The listing builds one solid part. Answer for the finished solid, in the listing's coordinates (mm). A direction names the side the tool comes from. Coordinates: 2 decimals unless noted, no trailing zeros. Loops run counter-clockwise (first coordinate to the right, second up) from the corner with the lowest first, then second, coordinate; pieces in that order, holes last. Notation, with made-up numbers: (78.25, 54) - (87.25, 54) arc R6 ccw to (87.25, 65) - close; hole circle Ø5 at (18.5, -35.75). An arc over 180 degrees is marked (long way). Return JSON: item names as keys, results as strings. Group by question number.
1. Section D-D (y = -12) is taken. Write down the section's boundary in (x, z).
2. Which of the six approach directions +Z, -Z, +X, -X, +Y, -Y give full straight-line access (tool end or side, diameter ignored) to faces 1 (the face through (23, -10, 12)), 2 (the face through (-20, -9, 36)), 3 (the face through (-23.04, 4.21, 38.35))?
3. The mould has two halves that part along Z. Classify faces 4 (the face through (-22.958, 12.843, 15.032)), 5 (the face through (0, -35, 3)), 6 (the face through (-22.958, 11.903, 34.802)), 7 (the face through (0, -10, 0)): pulls with the +Z half, pulls with the -Z half, needs draft (parallel to the pull), parting line crosses it, or undercut.
4. Section A-A (z = 25) is taken. Write down the section's boundary in (x, y), and give its area (3 significant figures).
5. Each of these flat-tipped pins is pushed along its axis until it touches: P1, Ø6.5, axis at x = 24, z = 27, coming from the -Y side; P2, Ø8, axis at y = -28, z = 13.5, coming from the +X side; P3, Ø1.8, axis at x = 22, y = -9.5, coming from the +Z side. Where does it stop, or does it pass through?
6. Section B-B (x = -21.5) is taken. Write down the section's boundary in (y, z).
7. Section C-C (z = 7) is taken. Write down the section's boundary in (x, y), and give its area (3 significant figures).
8. Find the intervals of material crossed by line 1 along Y through (x, z) = (-22.3, 37); line 2 along Y through (x, z) = (-22, 25); line 3 along Z through (x, y) = (-22.5, -12.5), in increasing order.
Autodesk Inventor part; units mm, degrees
ref_plane "YZ Plane" through (0, 0, 0) normal (1, 0, 0) x (0, 1, 0)
ref_plane "XZ Plane" through (0, 0, 0) normal (0, 1, 0) x (-1, 0, 0)
ref_plane "XY Plane" through (0, 0, 0) normal (0, 0, 1) x (1, 0, 0)
sketch "スケッチ1" plane through (0, 0, 0) normal (0, 0, 1) x (1, 0, 0)
  circle A0 centre (0, 0) radius 14
  line L0 (-12, -12) -> (12, -12)
  line L1 (12, -12) -> (12, 12)
  line L2 (12, 12) -> (-12, 12)
  line L3 (-12, 12) -> (-12, -12)
  line L4 (-12, -12) -> (12, 12) construction
  line L5 (12, -12) -> (-12, 12) construction
  circle A1 centre (-12, 12) radius 1.45
  circle A2 centre (12, 12) radius 1.45
  circle A3 centre (-12, -12) radius 1.45
  circle A4 centre (12, -12) radius 1.45
  line L6 (-20, -15) -> (20, -15)
  line L7 (20, -15) -> (20, 15)
  line L8 (20, 15) -> (-20, 15)
  line L9 (-20, 15) -> (-20, -15)
  line L10 (-20, -15) -> (20, 15) construction
  line L11 (20, -15) -> (-20, 15) construction
  dimension "d0" = 24
  dimension "d1" = 24
  dimension "d2" = 28
  dimension "d3" = 2.9
  dimension "d4" = 2.9
  dimension "d5" = 2.9
  dimension "d6" = 2.9
  dimension "d7" = 30
  dimension "d8" = 40
extrude "押し出し1" add sketch "スケッチ1" along normal blind 6 contours A0 L1 | L1 A0 L0 L3 L2 | A0 L2 A2 L1 | L1 A4 L0 A0 | L2 A0 | A2 L2 L1 | L1 L2 A2 | A0 L0 | A4 L0 L1 | L1 L0 A4 | A0 L3 A1 L2 | L0 A3 L3 A0 | L3 A0 | A1 L3 L2 | L2 L3 A1 | A3 L3 L0 | L0 L3 A3 | L9 L8 L7 L6
sketch "スケッチ3" plane through (0, 0, 0) normal (0, 0, -1) x (-1, 0, 0)
  line L0 (-20, -15) -> (-20, 15)
  line L1 (20, 15) -> (20, -15)
  line L2 (-20, 15) -> (-26, 15)
  line L3 (-26, 15) -> (-26, -15)
  line L4 (-26, -15) -> (-20, -15)
  line L5 (-20, -15) -> (-20, 15)
  line L6 (20, -15) -> (26, -15)
  line L7 (26, -15) -> (26, 15)
  line L8 (26, 15) -> (20, 15)
  line L9 (20, 15) -> (20, -15)
  dimension "d16" = 6
  dimension "d17" = 6
extrude "押し出し2" add sketch "スケッチ3" against normal blind 55
sketch "スケッチ7" plane through (-26, -15, 0) normal (0, -1, 0) x (1, 0, 0)
  line L0 (52, 0) -> (0, 0)
  line L1 (52, 0) -> (52, 55)
  line L2 (6, 6) -> (46, 6)
  line L3 (0, 0) -> (0, 55)
  line L4 (52, 0) -> (0, 0)
  line L5 (0, 0) -> (52, 0)
  line L6 (52, 0) -> (52, 6)
  line L7 (52, 6) -> (0, 6)
  line L8 (0, 6) -> (0, 0)
  point P0 (26, 0)
  point P1 (0, 6)
extrude "押し出し5" add sketch "スケッチ7" along normal blind 20
sketch "スケッチ8" plane through (0, 0, 0) normal (0, 0, -1) x (-1, 0, 0)
  line L0 (-26, 15) -> (26, 15)
  line L1 (26, -35) -> (26, 15)
  circle A0 centre (-1.5, -10.4) radius 25.65
  circle A1 centre (21.5, -30.4) radius 1.6
  circle A2 centre (-21.5, 7.6) radius 1.6
  point P0 (0, 0)
  dimension "d29" = 51.3
  dimension "d30" = 3.2
  dimension "d31" = 3.2
  dimension "d34" = 20
  dimension "d35" = 18
  dimension "d36" = 23
  dimension "d37" = 20
  dimension "d38" = 45.4
  dimension "d39" = 4.5
hole "穴1" at (-21.5, -30.4, 0) at (21.5, 7.6, 0) direction (0, 0, 1) diameter 4.4 depth 5
sketch "Sketch10" plane through (-26, -15, 55) normal (-1, 0, 0) x (0, 0, 1)
  line L0 (-55, -20) -> (-55, 30)
  line L1 (-49, -20) -> (-55, -20)
  line L2 (-49, 0) -> (-49, -20)
  line L3 (-49, 0) -> (0, 0)
  line L4 (0, 30) -> (0, 0)
  line L5 (-55, 30) -> (0, 30)
  circle A0 centre (-30, 15) radius 14
  point P0 (-55, 15)
  dimension "d58" = 28
  dimension "d59" = 15
  dimension "d60" = 25
extrude "Extrusion7" cut sketch "Sketch10" against normal blind 10 contours A0
sketch "Sketch11" plane through (-26, -15, 55) normal (-1, 0, 0) x (0, 0, 1)
  circle A0 centre (-30, 15) radius 14
  line L0 (-18, 27) -> (-42, 27)
  line L1 (-42, 27) -> (-42, 3)
  line L2 (-42, 3) -> (-18, 3)
  line L3 (-18, 3) -> (-18, 27)
  line L4 (-18, 27) -> (-42, 3) construction
  line L5 (-42, 27) -> (-18, 3) construction
  point P0 (-55, 15)
  dimension "d63" = 24
  dimension "d64" = 24
hole "Hole2" at (-26, -12, 37) at (-26, 12, 37) at (-26, 12, 13) at (-26, -12, 13) direction (1, 0, 0) diameter 4.4 depth 8.8 tip angle 118
sketch "スケッチ12" plane through (26, -15, 55) normal (1, 0, 0) x (0, 0, -1)
  line L0 (0, 0) -> (0, 30)
  line L1 (49, 0) -> (0, 0)
  line L2 (49, 0) -> (49, -20)
  line L3 (49, 0) -> (0, 0)
  line L4 (0, 0) -> (43, 0)
  line L5 (43, 0) -> (43, 10)
  line L6 (43, 10) -> (0, 10)
  line L7 (0, 10) -> (0, 0)
  point P0 (55, 15)
  point P1 (0, 10)
  dimension "d75" = 10
  dimension "d76" = 6
extrude "押し出し8" cut sketch "スケッチ12" against normal blind 10
sketch "スケッチ13" plane through (-26, -15, 6) normal (0, -1, 0) x (1, 0, 0)
  line L0 (0, 0) -> (6, 0)
  line L1 (6, 0) -> (6, 49)
  line L2 (0, 49) -> (6, 49)
  line L3 (0, 0) -> (0, 49)
  point P0 (26, -6)
extrude "押し出し9" add sketch "スケッチ13" along normal blind 10
properties part number "Print_Parts_H1"
The answers:
{
 "1": {"outline": "(-26, 0) - (26, 0) - (26, 12) - (20, 12) - (20, 6) - (-20, 6) - (-20, 10.8) - (-26, 10.8) - close; (-26, 15.2) - (-20, 15.2) - (-20, 17.79) - (-26, 17.79) - close; (-26, 32.21) - (-20, 32.21) - (-20, 34.8) - (-26, 34.8) - close; (-26, 39.2) - (-20, 39.2) - (-20, 55) - (-26, 55) - close"},
 "2": {"face 1": "+Z, +X, -Y", "face 2": "+Z, +Y, -Y", "face 3": "-X"},
 "3": {"face 4": "undercut", "face 5": "needs draft", "face 6": "undercut", "face 7": "pulls with the -Z half"},
 "4": {"outline": "(-26, -25) - (-20, -25) - (-20, -14) - (-26, -14) - close; (-26, 14) - (-20, 14) - (-20, 15) - (-26, 15) - close; (20, -5) - (26, -5) - (26, 15) - (20, 15) - close", "area": "192 mm2"},
 "5": {"P1": "stops at y = -5", "P2": "stops at x = -20", "P3": "stops at z = 12"},
 "6": {"outline": "(-35, 0) - (-32.6, 0) - (-32.6, 5) - (-28.2, 5) - (-28.2, 0) - (15, 0) - (15, 55) - (-25, 55) - (-25, 6) - (-35, 6) - close; hole circle Ø4.4 at (-12, 13); hole circle Ø4.4 at (-12, 37); hole circle Ø28 at (0, 25); hole circle Ø4.4 at (12, 13); hole circle Ø4.4 at (12, 37)"},
 "7": {"outline": "(-26, -25) - (-20, -25) - (-20, 15) - (-26, 15) - close; (20, -15) - (26, -15) - (26, 15) - (20, 15) - close", "area": "420 mm2"},
 "8": {"line 1": "y = -25 to -14.2, -9.8 to -7.21, 7.21 to 9.8, 14.2 to 15", "line 2": "y = -25 to -14, 14 to 15", "line 3": "z = 0 to 10.86, 15.14 to 18.7, 31.3 to 34.86, 39.14 to 55"}
}
